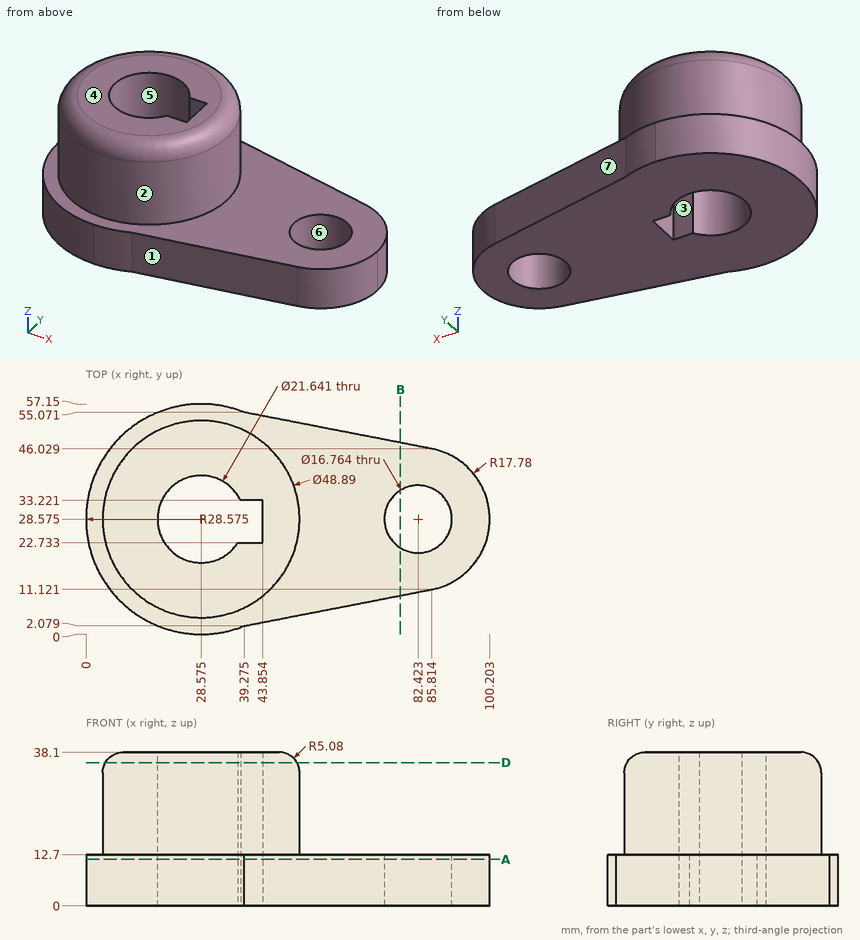
The figure shows three views and two pictorial views of one solid part (mm, origin at its lowest corner). Answer the questions. A direction names the side the tool comes from. Give positions to 0.01 mm unless a question says otherwise; leave off trailing zeros. Order: outer loops, then holes, each group sorted by start corner. A loop starts at its lowest first (then second) coordinate and runs counter-clockwise, first axis right, second up. Notation, with made-up numbers: M 31.25,12.5 L 82.25,12.5 A13 ccw 82.25,23.5 Z; hole C 74,-1.5 d4. An arc over 180 degrees is marked long. Return JSON: item names as keys, results as strings.
Q1. Which of the six approach directions +Z, -Z, +X, -X, +Y, -Y give full straight-line access (tool end or side, diameter ignored) to the marked faces 1, 2 and 3?
Answer below:
{"face 1": "+Z, -Z, +X, -Y", "face 2": "+Z", "face 3": "+Z, -Z"}
Q2. Find section B-B, the plane x = 78. Write down the section's boundary in (y, z) (1 decimal), and give its area (3 significant figures).
Answer below:
{"outline": "M 9.6,0 L 21.5,0 L 21.5,12.7 L 9.6,12.7 Z; M 35.7,0 L 47.5,0 L 47.5,12.7 L 35.7,12.7 Z", "area": "301 mm^2"}
Q3. Find section D-D, the plane z = 35.5. Write down the section's boundary in (x, y) (1 decimal), and give its area (3 significant figures).
Answer below:
{"outline": "C 28.6,28.6 d47.6; hole M 37.7,22.7 L 43.9,22.7 L 43.9,33.2 L 38.3,33.2 A10.8 ccw long Z", "area": "1,360 mm^2"}
Q4. Find section A-A, the plane z = 11.5. State how many separate pieces and enclosed holes the cut face has, and give its area (3 significant figures).
Answer below:
{"separate pieces": "1", "enclosed holes": "2", "area": "3,660 mm^2"}
Q5. The mould has two halves that part along X. Classify the marked faces 4, 5, 6 and 7: pulls with the +X half, pulls with the -X half, needs draft (parallel to the pull), parting line crosses it, or undercut.
Answer below:
{"face 4": "needs draft", "face 5": "undercut", "face 6": "undercut", "face 7": "pulls with the +X half"}
Q6. Each of these flat-tipped pins is pushed along its axis until it touches: pin 1 (4 mm diameter, centred on x = 23, z = 5.5, fed in from -Y) (1 decimal); pin 2 (1.9 mm diameter, centred on x = 42, z = 20.5, fed in from +Y); pin 3 (5 mm diameter, centred on x = 64, y = 47.5, fed in from +Z). Where does it stop, or does it pass through?
Answer below:
{"pin 1": "stops at y = 0.2", "pin 2": "stops at y = 49.6", "pin 3": "stops at z = 12.7"}
Q7. Find the intervals of material crossed by line 1 along X through (y, z) = (29.5, 6.5) (1 decimal); line 2 along Z through (x, y) = (10.5, 49.5); line 3 along X through (y, z) = (50.5, 32) (1 decimal), in increasing order. Write a range as [from, to].
Answer below:
{"line 1": "x = [0, 17.8], [43.9, 74.1], [90.8, 100.2]", "line 2": "z = [0, 12.7]", "line 3": "x = [17.8, 39.4]"}
